Autodesk Inventor part; units mm, degrees
ref_plane "YZ Plane" through (0, 0, 0) normal (1, 0, 0) x (0, 1, 0)
ref_plane "XZ Plane" through (0, 0, 0) normal (0, 1, 0) x (-1, 0, 0)
ref_plane "XY Plane" through (0, 0, 0) normal (0, 0, 1) x (1, 0, 0)
sketch "スケッチ1" plane through (0, 0, 0) normal (0, 1, 0) x (-1, 0, 0)
  line L0 (7.6573, 10.2043) -> (-8.8427, 10.2043)
  line L1 (-8.8427, 10.2043) -> (-8.8427, -15.9957)
  line L2 (-8.8427, -15.9957) -> (7.6573, -15.9957)
  line L3 (7.6573, -15.9957) -> (7.6573, 10.2043)
  line L4 (5.6573, 8.2043) -> (-6.8427, 8.2043)
  line L5 (-6.8427, 8.2043) -> (-6.8427, -13.9957)
  line L6 (-6.8427, -13.9957) -> (5.6573, -13.9957)
  line L7 (5.6573, -13.9957) -> (5.6573, 8.2043)
  line L8 (5.6573, 8.2043) -> (0.5388, 8.2043)
  line L9 (0.5388, -13.9957) -> (5.6573, -13.9957)
  line L10 (5.6573, -13.9957) -> (5.6573, 8.2043)
  circle A0 centre (-0.5927, -2.8957) radius 2.5
  line L11 (-6.8427, 4.5043) -> (5.6573, 4.5043)
  line L12 (5.6573, 4.5043) -> (5.6573, 1.5043)
  line L13 (5.6573, 1.5043) -> (-6.8427, 1.5043)
  line L14 (-6.8427, 1.5043) -> (-6.8427, 4.5043)
  point P0 (0, 0)
  dimension "d0" = 12.5
  dimension "d1" = 22.2
  dimension "d2" = 2
  dimension "d3" = 2
  dimension "d4" = 2
  dimension "d5" = 2
  dimension "d6" = 3.7
  dimension "d7" = 3
  dimension "d8" = 5
  dimension "d9" = 6.25
  dimension "d11" = 13.1
  dimension "d12" = 13.1
  dimension "d17" = 6.25
extrude "押し出し1" add sketch "スケッチ1" along normal blind 5 contours L3 L2 L1 L0
extrude "押し出し2" add sketch "スケッチ1" against normal blind 5 contours L3 L2 L1 L0 | L7 L11 L5 L4 | L7 L6 L5 L13
sketch "スケッチ2" plane through (0, 5, 0) normal (0, 1, 0) x (1, 0, 0)
  line L0 (8.8427, -10.2043) -> (8.8427, 15.9957)
  line L1 (8.8427, 15.9957) -> (-7.6728, 15.9957)
  line L2 (-7.6728, 15.9957) -> (-7.6728, 14.001)
  line L3 (-7.6728, 14.001) -> (8.8427, 14.001)
  line L4 (8.8427, 14.001) -> (8.8427, 15.9957)
  point P0 (0, 0)
properties part number "armpart3"
Could you check a few things on this model? Use its own coordinates, in mm. A direction names the side the tool comes from. Give positions to 0.01 mm unless a question says otherwise; leave off trailing zeros. Order: outer loops, then holes, each group sorted by start corner. A loop starts at its lowest first (then second) coordinate and runs counter-clockwise, first axis right, second up.
Q1. I'm going to push flat-ended pins straight in: P1, Ø1, axis at x = -0.5, z = -4, coming from the -Y side; P2, Ø4, axis at x = 2.5, z = 6, coming from the +Y side. Where does each tip first touch, or does it pass through?
Q2. Suppose I cut it at B-B, the plane y = 1.75. Write out the boundary of the cut face in (x, z), and give its area (3 significant figures).
Q3. Suppose I cut it at A-A, the plane x = -2.5. Write out the boundary of the cut face in (y, z), and give its area (3 significant figures).
Q4. We'd pull the mould along X, two halves only. Please class faces 4 (the flat face through (1, -2, 1.504)), 5 (the flat face through (-7.657, 0, -3)), 6 (the flat face through (1, -5, -6)): +X half, -X half, draft (parallel to the pull), parting line (faces both ways), or undercut.
Q5. Suppose I cut it at D-D, the plane z = -6. Write out the boundary of the cut face in (x, y), and give its area (4 significant figures).
Q6. If I drill on line 1 along X through (y, z) = (-0.5, 3); line 2 along Z through (x, y) = (5, -1); line 3 along Z through (x, y) = (3, 0.75), over which ranges is the centre line in solid material (lowest first)?
Q7. Suppose I cut it at C-C, the plane x = -0.5. Write out the boundary of the cut face in (y, z).
Q8. For faces 1 (the flat face through (1, 0, 6)), 2 (the flat face through (1, -2, 4.504)), 3 (the flat face through (0, 0, 10.204)), which set-ups out of +Z, -Z, +X, -X, +Y, -Y let a thin tool reach every point of the face, with its end or its side?
Solution:
1. P1: passes through
1. P2: stops at y = 0
2. outline: (-7.66, -16) - (8.84, -16) - (8.84, 10.2) - (-7.66, 10.2) - close; hole (-5.66, -14) - (6.84, -14) - (6.84, 8.2) - (-5.66, 8.2) - close
2. area: 155 mm2
3. outline: (-5, -16) - (5, -16) - (5, -14) - (0, -14) - (0, 1.5) - (-5, 1.5) - close; (-5, 4.5) - (0, 4.5) - (0, 8.2) - (5, 8.2) - (5, 10.2) - (-5, 10.2) - close
3. area: 136 mm2
4. face 4: undercut
4. face 5: -X half
4. face 6: draft
5. outline: (-7.66, -5) - (8.84, -5) - (8.84, 5) - (6.84, 5) - (6.84, 0) - (-5.66, 0) - (-5.66, 5) - (-7.66, 5) - close
5. area: 102.5 mm2
6. line 1: x = -7.66 to -5.66, 6.84 to 8.84
6. line 2: z = -16 to 1.5, 4.5 to 10.2
6. line 3: z = -16 to -14, 8.2 to 10.2
7. outline: (-5, -16) - (5, -16) - (5, -14) - (0, -14) - (0, -5.14) - (-5, -5.14) - close; (-5, -0.65) - (0, -0.65) - (0, 1.5) - (-5, 1.5) - close; (-5, 4.5) - (0, 4.5) - (0, 8.2) - (5, 8.2) - (5, 10.2) - (-5, 10.2) - close
8. face 1: +Y
8. face 2: +Y, -Y
8. face 3: +Z, +X, -X, +Y, -Y
